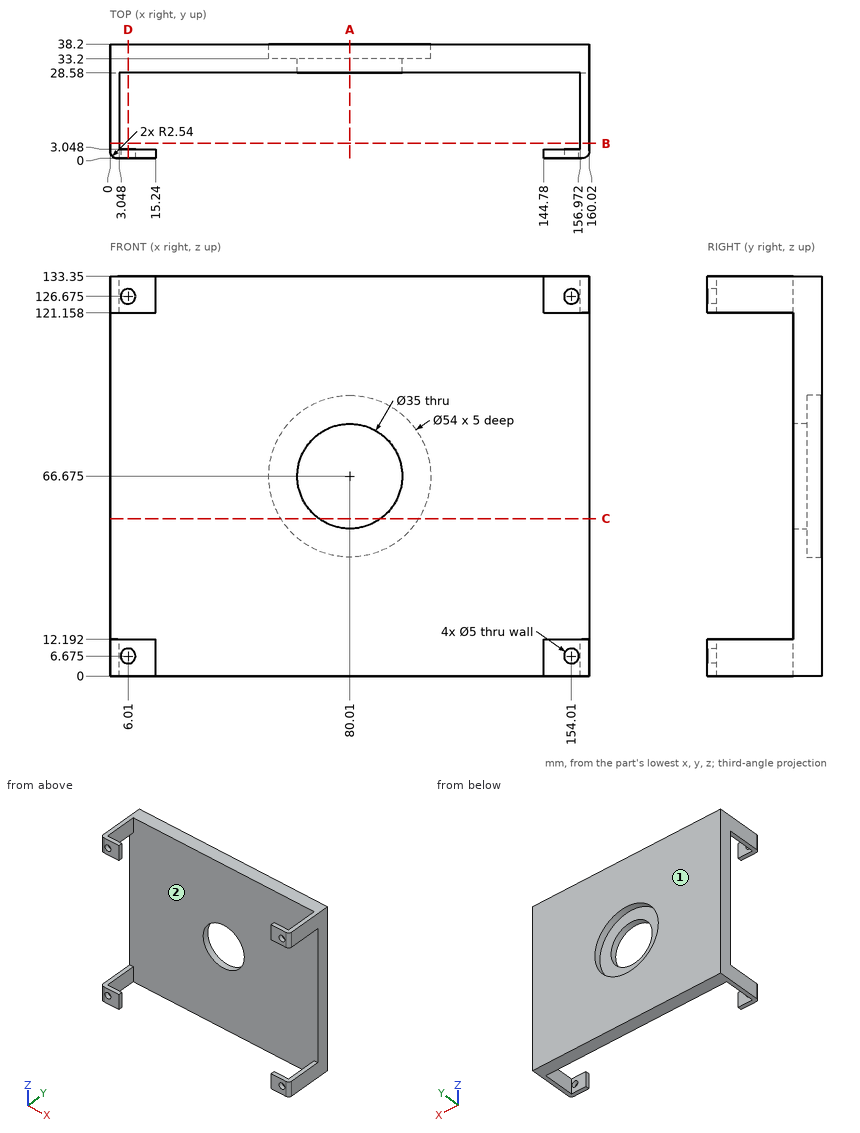
Can you work these out from the drawing? Everything is in mm from the part's minimum corner. Round coordinates to 2 decimals unless told otherwise and drop trailing zeros. Write each loop counter-clockwise with the first axis right and the second up, starting at its lowest first coordinate (ties: lowest second). Pieces come first, ordered by that corner, then holes.
1. Suppose I cut it at B-B (y = 5). List the corners of the cut face in (x, z) for me, and give its area (3 significant figures).
2. Will these pins go through, and if not, where does the flat tip stop? pin 1 Ø1.5 at (y, z) = (34, 100) entering from -X; pin 2 Ø2 at (x, z) = (38, 116) entering from -Y; pin 3 Ø12 at (x, y) = (110, 20) entering from +Z; pin 4 Ø0.9 at (y, z) = (1.5, 125.5) entering from -X.
3. Suppose I cut it at C-C (z = 52.5). List the corners of the cut face in (x, y) for me, and give its area (3 significant figures).
4. If we mould it in two halves opening along X, with no side actions, what happens to the marked faces 1 and 2? For each: released by +X, released by -X, zero draft, split by the parting line, or undercut.
5. Suppose I cut it at A-A (x = 80.01). List the corners of the cut face in (y, z) for me (3 decimals), and give its area (3 significant figures).
6. Suppose I cut it at D-D (x = 6.01). List the corners of the cut face in (y, z) for me (3 decimals).
7. I need wall thicknesses on L1, parallel to Z at x = 6, y = 1; L2, parallel to Y at x = 145, z = 10; L3, parallel to Z at x = 149, y = 2.5. Which ranges of each line are inside material? Lowest first, please.
Answer sheet:
1. outline: (0, 0) - (3.05, 0) - (3.05, 12.19) - (0, 12.19) - close; (0, 121.16) - (3.05, 121.16) - (3.05, 133.35) - (0, 133.35) - close; (156.97, 0) - (160.02, 0) - (160.02, 12.19) - (156.97, 12.19) - close; (156.97, 121.16) - (160.02, 121.16) - (160.02, 133.35) - (156.97, 133.35) - close
1. area: 149 mm2
2. pin 1: stops at x = 0
2. pin 2: stops at y = 28.58
2. pin 3: passes through
2. pin 4: stops at x = 0.07
3. outline: (0, 28.58) - (69.75, 28.58) - (69.75, 33.2) - (57.03, 33.2) - (57.03, 38.2) - (0, 38.2) - close; (90.27, 28.58) - (160.02, 28.58) - (160.02, 38.2) - (102.99, 38.2) - (102.99, 33.2) - (90.27, 33.2) - close
3. area: 1,210 mm2
4. face 1: zero draft
4. face 2: undercut
5. outline: (28.58, 0) - (38.2, 0) - (38.2, 39.675) - (33.2, 39.675) - (33.2, 49.175) - (28.58, 49.175) - close; (28.58, 84.175) - (33.2, 84.175) - (33.2, 93.675) - (38.2, 93.675) - (38.2, 133.35) - (28.58, 133.35) - close
5. area: 851 mm2
6. outline: (0, 0) - (3.048, 0) - (3.048, 4.175) - (0, 4.175) - close; (0, 9.175) - (3.048, 9.175) - (3.048, 12.192) - (0, 12.192) - close; (0, 121.158) - (3.048, 121.158) - (3.048, 124.175) - (0, 124.175) - close; (0, 129.175) - (3.048, 129.175) - (3.048, 133.35) - (0, 133.35) - close; (28.58, 0) - (38.2, 0) - (38.2, 133.35) - (28.58, 133.35) - close
7. L1: z = 0 to 4.18, 9.17 to 12.19, 121.16 to 124.18, 129.17 to 133.35
7. L2: y = 0 to 3.05, 28.58 to 38.2
7. L3: z = 0 to 12.19, 121.16 to 133.35
